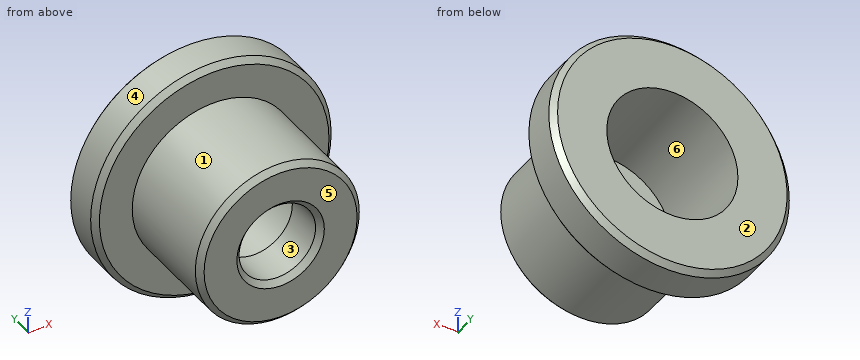
from build123d import *

# Parameters (mm, degrees)
F0_R     = 11
F1_DEPTH = 4
F2_R     = 7.5
F5_DEPTH = 10
F3_R     = 6
F6_DEPTH = 10
F7_R     = 3.5
F4_DEPTH = 25
F8_SIZE  = 0.5


with BuildPart() as f1:
    # F0 (on Front) → F1 (new body)
    with BuildSketch(Plane.XZ):
        Circle(F0_R)
    extrude(amount=F1_DEPTH)

    # F2 (on face) → F5 (join)
    with BuildSketch(Plane.XZ.offset(4)):
        Circle(F2_R)
    extrude(amount=F5_DEPTH)

    # F3 (on face) → F6 (cut)
    with BuildSketch(Plane(origin=(0, 0, 0), x_dir=(-1, 0, 0), z_dir=(0, 1, 0))):
        Circle(F3_R)
    extrude(amount=-F6_DEPTH, mode=Mode.SUBTRACT)

    # F7 (on face) → F4 (cut)
    with BuildSketch(Plane.XZ.offset(14)):
        Circle(F7_R)
    extrude(amount=-F4_DEPTH, mode=Mode.SUBTRACT)

    # F8
    f8_edges = [f1.edges().sort_by_distance(p)[0] for p in [
        (-7.5, -14, 0),
        (-3.5, -14, 0),
        (11, -2, 0),
        (-11, 0, 0),
        (-11, -4, 0),
    ]]
    chamfer(f8_edges, length=F8_SIZE)


solid = f1.part
Input: part model. Units: mm. Frame: model coordinates. Face numbers are marked on the shaded views. A direction names the side the tool comes from. Coordinates: 2 decimals unless noted, no trailing zeros. Loops run counter-clockwise (first coordinate to the right, second up) from the corner with the lowest first, then second, coordinate; pieces in that order, holes last. Notation, with made-up numbers: (77, 15.5) - (94, 15.5) arc R13 ccw to (94, 29.5) - close; hole circle Ø3 at (41, -38.5). An arc over 180 degrees is marked (long way). Answer in a Markdown table with one row per item. Add a question column.
Item 1: Access query for the marked faces 1 and 2. Directions: +Z, -Z, +X, -X, +Y, -Y. A direction counts if a zero-diameter tool reaches every point of the face in a straight line with its end or side. Return the directions, or none.
Item 2: Section query A-A on x = 0. Return the cut outline in (y, z), then the cut area to 3 significant figures.
Item 3: Section query C-C on y = -11.5. Return the cut outline in (x, z), then the cut area to 3 significant figures.
Item 4: Section query B-B on z = 0. Return the cut outline in (x, y).
Item 5: Section query D-D on y = -3. Return the cut outline in (x, z), then the cut area to 3 significant figures.
Item 6: Contact query for flat-ended pins moving along their axis: P1, Ø2, axis at x = 2, y = -2.5, coming from the -Z side; P2, Ø8, axis at y = -5.5, z = 4, coming from the +X side; P3, Ø6, axis at x = 2.5, z = -1.5, coming from the +Y side. Output: stop coordinate, or through.
Item 7: Mould query, pull axis Z, two halves, no side actions, for the marked faces 3, 4, 5 and 6. Classes: released by +Z, released by -Z, zero draft, split by the parting line, or undercut.
Item 8: Line query: line 1 along Z through (x, y) = (0, -10.8); line 2 along Z through (x, y) = (0, -6.75); line 3 along Y through (x, z) = (-7.5, -6.5). Output: solid intervals per line, ascending. Write a range as [from, to].
Recorded:
| question | item | result |
|---|---|---|
| 1 | face 1 | -Y |
| 1 | face 2 | +Z, -Z, +X, -X, +Y |
| 2 | outline | (-14, -7) - (-13.5, -7.5) - (-4, -7.5) - (-4, -10.5) - (-3.5, -11) - (-0.5, -11) - (0, -10.5) - (0, -6) - (-10, -6) - (-10, -3.5) - (-13.5, -3.5) - (-14, -4) - close; (-14, 4) - (-13.5, 3.5) - (-10, 3.5) - (-10, 6) - (0, 6) - (0, 10.5) - (-0.5, 11) - (-3.5, 11) - (-4, 10.5) - (-4, 7.5) - (-13.5, 7.5) - (-14, 7) - close |
| 2 | area | 89.0 mm^2 |
| 3 | outline | circle Ø15 at (0, 0); hole circle Ø7 at (0, 0) |
| 3 | area | 138 mm^2 |
| 4 | outline | (-11, -3.5) - (-10.5, -4) - (-7.5, -4) - (-7.5, -13.5) - (-7, -14) - (-4, -14) - (-3.5, -13.5) - (-3.5, -10) - (-6, -10) - (-6, 0) - (-10.5, 0) - (-11, -0.5) - close; (3.5, -13.5) - (4, -14) - (7, -14) - (7.5, -13.5) - (7.5, -4) - (10.5, -4) - (11, -3.5) - (11, -0.5) - (10.5, 0) - (6, 0) - (6, -10) - (3.5, -10) - close |
| 5 | outline | circle Ø22 at (0, 0); hole circle Ø12 at (0, 0) |
| 5 | area | 267 mm^2 |
| 6 | P1 | z = -10.95 |
| 6 | P2 | x = 10.99 |
| 6 | P3 | y = -10 |
| 7 | face 3 | undercut |
| 7 | face 4 | split by the parting line |
| 7 | face 5 | zero draft |
| 7 | face 6 | undercut |
| 8 | line 1 | [-7.5, -3.5], [3.5, 7.5] |
| 8 | line 2 | [-7.5, -6], [6, 7.5] |
| 8 | line 3 | [-4, 0] |
